Answer from the drawing. Dimensions are ordinates in mm from the lowest x, y and z of the part. A direction names the side the tool comes from. Round coordinates to 2 decimals unless told otherwise and drop trailing zeros. Loops run counter-clockwise (first coordinate to the right, second up) from the corner with the lowest first, then second, coordinate; pieces in that order, holes last. Notation, with made-up numbers: (33.5, -3) - (59.5, -3) arc R6 cw to (59.5, 8) - close; hole circle Ø6 at (-2, 41.5). An arc over 180 degrees is marked (long way). Return JSON: item names as keys, results as strings.
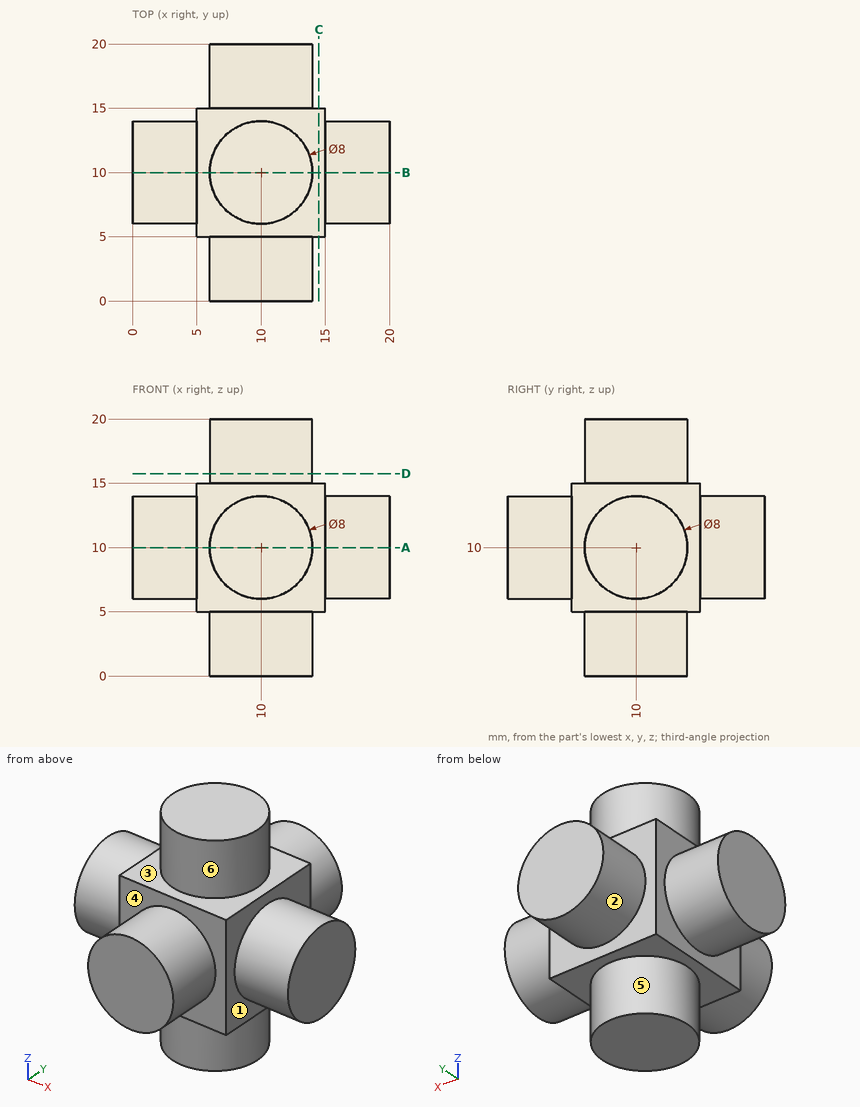
1) Section C-C (x = 14.5) is taken. Give the vertices of the cut face in (y, z).
Verdict:
{"outline": "(5, 5) - (15, 5) - (15, 15) - (5, 15) - close"}
2) Find the intervals of material crossed by L1, parallel to X at y = 7.25, z = 14.5; L2, parallel to X at y = 1, z = 9; L3, parallel to Z at x = 10.75, y = 2.25, in increasing order.
Verdict:
{"L1": "x = 5 to 15", "L2": "x = 6.13 to 13.87", "L3": "z = 6.07 to 13.93"}
3) Flat-ended cylindrical pins translate along their axes: pin 1 (5 mm diameter, centred on x = 2, z = 11.5, fed in from +Y); pin 2 (2 mm diameter, centred on y = 3, z = 14, fed in from -X); pin 3 (1.5 mm diameter, centred on y = 16, z = 6, fed in from +X). Find the tip coordinate at first contact, or state that the pin passes through.
Verdict:
{"pin 1": "stops at y = 14", "pin 2": "stops at x = 7.35", "pin 3": "stops at x = 12.33"}
4) Section A-A (z = 10) is taken. Give the vertices of the cut face in (x, y).
Verdict:
{"outline": "(0, 6) - (5, 6) - (5, 5) - (6, 5) - (6, 0) - (14, 0) - (14, 5) - (15, 5) - (15, 6) - (20, 6) - (20, 14) - (15, 14) - (15, 15) - (14, 15) - (14, 20) - (6, 20) - (6, 15) - (5, 15) - (5, 14) - (0, 14) - close"}
5) A tool of negligible diameter and unlimited length cuts with its end or side. For the marked faces 4, 5 and 6, from which of +Z, -Z, +X, -X, +Y, -Y can it reach the whole face along a straight path? Write none if from no direction.
Verdict:
{"face 4": "-Y", "face 5": "-Z", "face 6": "+Z"}
6) Section D-D (z = 15.75) is taken. Give the vertices of the cut face in (x, y), and give its area (3 significant figures).
Verdict:
{"outline": "circle Ø8 at (10, 10)", "area": "50.3 mm2"}
7) Determine the mould class of the marked faces 1, 2 and 3 for opening direction X: pulls with the +X half, pulls with the -X half, needs draft (parallel to the pull), parting line crosses it, or undercut.
Verdict:
{"face 1": "pulls with the +X half", "face 2": "parting line crosses it", "face 3": "needs draft"}
